Autodesk Inventor part; units mm, degrees
ref_plane "YZ Plane" through (0, 0, 0) normal (1, 0, 0) x (0, 1, 0)
ref_plane "XZ Plane" through (0, 0, 0) normal (0, 1, 0) x (-1, 0, 0)
ref_plane "XY Plane" through (0, 0, 0) normal (0, 0, 1) x (1, 0, 0)
sketch "Sketch1" plane through (0, 0, 0) normal (0, 0, 1) x (1, 0, 0)
  line L0 (-6.25, 6.25) -> (6.25, 6.25)
  line L1 (6.25, 6.25) -> (6.25, -6.25)
  line L2 (6.25, -6.25) -> (-6.25, -6.25)
  line L3 (-6.25, -6.25) -> (-6.25, 6.25)
  line L4 (-10, 10) -> (10, 10)
  line L5 (10, 10) -> (10, -10)
  line L6 (10, -10) -> (-10, -10)
  line L7 (-10, -10) -> (-10, 10)
  line L8 (-10, 10) -> (10, -10) construction
  line L9 (10, 10) -> (-10, -10) construction
  dimension "d3" = 20
  dimension "d4" = 20
  dimension "d5" = 3.75
  dimension "d6" = 16.25
  dimension "d7" = 3.75
  dimension "d8" = 16.25
extrude "Extrusion1" add sketch "Sketch1" along normal blind 55
sketch "Sketch2" plane through (0, 0, 55) normal (0, 0, 1) x (1, 0, 0)
  line L0 (10, 10) -> (-10, 10)
  line L1 (-10, -10) -> (10, -10)
  line L2 (10, -10) -> (10, 10)
  line L3 (10, 10) -> (-10, 10)
  line L4 (-10, 10) -> (-10, -10)
  line L5 (-10, -10) -> (10, 10) construction
  line L6 (10, -10) -> (-10, 10) construction
  point P0 (0, 0)
extrude "Extrusion2" add sketch "Sketch2" along normal blind 3
sketch "Sketch3" plane through (0, 0, 55) normal (0, 0, -1) x (-1, 0, 0)
  circle A0 centre (0, 0) radius 4
  dimension "d13" = 8
extrude "Extrusion3" add sketch "Sketch3" along normal blind 14
sketch "Sketch4" plane through (10, -10, 0) normal (1, 0, 0) x (0, 0, -1)
  line L0 (0, 0) -> (-58, 0)
  line L1 (0, 0) -> (-10, 0)
  line L2 (-10, 0) -> (-10, 3)
  line L3 (-10, 3) -> (0, 3)
  line L4 (0, 3) -> (0, 0)
  line L5 (-58, 0) -> (-58, 20)
  line L6 (-58, 0) -> (-48, 0)
  line L7 (-48, 0) -> (-48, 3)
  line L8 (-48, 3) -> (-58, 3)
  line L9 (-58, 3) -> (-58, 0)
  point P0 (0, 10)
  dimension "d16" = 10
  dimension "d17" = 3
  dimension "d18" = 10
  dimension "d19" = 3
extrude "Extrusion4" add sketch "Sketch4" along normal blind 10
sketch "Sketch5" plane through (-10, -10, 0) normal (-1, 0, 0) x (0, 0, 1)
  line L0 (0, 0) -> (0, 20)
  line L1 (0, 3) -> (10, 3)
  line L2 (0, 0) -> (10, 0)
  line L3 (10, 0) -> (10, 3)
  line L4 (10, 3) -> (0, 3)
  line L5 (0, 3) -> (0, 0)
  line L6 (58, 20) -> (58, 0)
  line L7 (58, 0) -> (48, 0)
  line L8 (48, 0) -> (48, 3)
  line L9 (48, 3) -> (58, 3)
  line L10 (58, 3) -> (58, 0)
  point P0 (0, 10)
  dimension "d22" = 10
  dimension "d23" = 3
  dimension "d24" = 10
  dimension "d25" = 3
extrude "Extrusion5" add sketch "Sketch5" along normal blind 10
fillet "Fillet1" radius 5 12 edges at (-20, -8.5, 10) (-20, -8.5, 0) (-10, -8.5, 10) (-10, -8.5, 48) (-20, -8.5, 48) (-20, -8.5, 58) (20, -8.5, 0) (10, -8.5, 10) (20, -8.5, 10) (10, -8.5, 48) (20, -8.5, 48) (20, -8.5, 58)
sketch "Sketch6" plane through (10, -7, 15) normal (0, 1, 0) x (1, 0, 0)
  arc A0 (-25, 15) -> (-25, 5) centre (-25, 10) ccw
  circle A1 centre (-25, 10) radius 2
  arc A2 (5, 5) -> (5, 15) centre (5, 10) ccw
  circle A3 centre (5, 10) radius 2
  arc A4 (-25, -33) -> (-25, -43) centre (-25, -38) ccw
  circle A5 centre (-25, -38) radius 2
  arc A6 (5, -43) -> (5, -33) centre (5, -38) ccw
  circle A7 centre (5, -38) radius 2
  point P0 (-10, 15)
  dimension "d29" = 4
  dimension "d30" = 4
  dimension "d31" = 4
extrude "Extrusion6" cut sketch "Sketch6" against normal blind 10
fillet "Fillet2" radius 5 2 edges at (-10, 10, 29) (10, 10, 29)
sketch "Sketch7" plane through (-5, 10, 0) normal (0, 1, 0) x (1, 0, 0)
  arc A0 (7.7, -10) -> (2.3, -10) centre (5, -10) ccw
  line L0 (0, -58) -> (0, 0)
  arc A1 (2.3, -14.35) -> (7.7, -14.35) centre (5, -14.35) ccw
  line L1 (2.3, -14.35) -> (2.3, -10)
  line L2 (7.7, -14.35) -> (7.7, -10)
  point P0 (5, 0)
  dimension "d35" = 5.4
  dimension "d36" = 5
  dimension "d37" = 10
  dimension "d38" = 5.4
  dimension "d39" = 4.35
  dimension "d40" = 5
extrude "Extrusion7" cut sketch "Sketch7" against normal blind 10
sketch "Sketch8" plane through (-5, 10, 0) normal (0, 1, 0) x (1, 0, 0)
  line L0 (2.3, -10) -> (2.3, -14.35)
  line L1 (2.3, -12.175) -> (-5, -12.175)
  line L2 (-5, 0) -> (-5, -58)
  arc A0 (-5, -15) -> (-10, -10) centre (-10, -15) ccw
  line L3 (-5, -12.175) -> (-5, -15)
  line L4 (-5, -15) -> (-18.139, -15)
  line L5 (-18.139, -15) -> (-18.139, 3.699)
  line L6 (-18.139, 3.699) -> (27.6458, 3.699)
  line L7 (27.6458, 3.699) -> (27.6458, -15)
  line L8 (15, -15) -> (15, -43)
  line L9 (27.6458, -15) -> (15, -15)
  line L10 (15, -15) -> (15, -12.175)
  arc A1 (20, -10) -> (15, -15) centre (20, -15) ccw
  line L11 (15, -12.175) -> (2.3, -12.175)
  point P0 (5, 0)
  dimension "d43" = 12.6458
  dimension "d44" = 33.139
  dimension "d45" = 18.699
extrude "Extrusion8" cut sketch "Sketch8" against normal blind 20
sketch "Sketch9" plane through (-2.7, 10, 12.175) normal (0, 0, -1) x (-1, 0, 0)
  circle A0 centre (-10.825, -10) radius 0.925
  circle A1 centre (-2.7, -18.125) radius 0.925
  circle A2 centre (5.425, -10) radius 0.925
  line L0 (-12.7, -20) -> (-12.7, -5)
  line L1 (7.3, -20) -> (-12.7, -20)
  line L2 (3.55, -16.25) -> (3.55, -3.75)
  point P0 (-2.7, -10)
  dimension "d48" = 1.85
  dimension "d49" = 1.85
  dimension "d50" = 1.85
  dimension "d51" = 1.875
  dimension "d52" = 1.875
  dimension "d53" = 1.875
  dimension "d54" = 0
  dimension "d55" = 0
  dimension "d56" = 0
extrude "Extrusion9" cut sketch "Sketch9" against normal blind 5
properties part number "14 slot pinhuls groot"
The model under review builds one solid part; all positions refer to its coordinate system, in mm. A direction names the side the tool comes from. Round coordinates to 2 decimals unless told otherwise and drop trailing zeros. Loops run counter-clockwise (first coordinate to the right, second up) from the corner with the lowest first, then second, coordinate; pieces in that order, holes last. Notation, with made-up numbers: (-24, -39.75) -> (-1, -39.75) arc R20 cw to (-1, -13.75) -> close; hole circle Ø7 at (56.25, -39). An arc over 180 degrees is marked (long way). Return JSON: item names as keys, results as strings.
(1) For faces 4 (the flat face through (10, -2, 35)), 5 (the flat face through (2.7, 8, 13)), 6 (the cylindrical face through (-8, 9, 35)), 7 (the flat face through (0, -8, 17.175)), list the 3-axis set-ups (+Z, -Z, +X, -X, +Y, -Y) from which the entire face can be reached by the end or side of a thin tool; tool diameter is ignored.
Solved:
{"face 4": "-Z, +X, +Y", "face 5": "-Z, +Y", "face 6": "+Z, -Z, -X, +Y", "face 7": "-Z"}
(2) For pin 1 (5 mm diameter, centred on x = 17, z = 52.5, fed in from +Y); pin 2 (1 mm diameter, centred on y = 3.5, z = 24.5, fed in from -X); pin 3 (2.5 mm diameter, centred on y = 8.5, z = 13, fed in from +X), all flat-tipped, find the tip position at first contact; note any pin that passes through.
Solved:
{"pin 1": "y = -7", "pin 2": "x = -10", "pin 3": "x = 9.47"}
(3) The part is to be moulded in two halves that separate along Y. For faces 1 (the flat face through (13, -7, 52)), 2 (the flat face through (0, 6.25, 33)), 3 (the flat face through (-10, -3, 35)), say which applies: released by +Y, released by -Y, zero draft, split by the parting line, or undercut.
Solved:
{"face 1": "released by +Y", "face 2": "undercut", "face 3": "zero draft"}
(4) Add section A-A on z = 34.5. Write out the cut boundary in (x, y), plus the area to 3 significant figures.
Solved:
{"outline": "(-10, -10) -> (10, -10) -> (10, 5) arc R5 ccw to (5, 10) -> (-5, 10) arc R5 ccw to (-10, 5) -> close; hole (-6.25, -6.25) -> (6.25, -6.25) -> (6.25, 6.25) -> (-6.25, 6.25) -> close", "area": "233 mm2"}
(5) Add section D-D on y = -3. Write out the cut boundary in (x, z) (3 decimals), plus the area to 3 significant figures.
Solved:
{"outline": "(-10, 12.175) -> (-6.25, 12.175) -> (-6.25, 55) -> (-2.646, 55) -> (-2.646, 41) -> (2.646, 41) -> (2.646, 55) -> (6.25, 55) -> (6.25, 12.175) -> (10, 12.175) -> (10, 58) -> (-10, 58) -> close", "area": "455 mm2"}
(6) For line 1 (X direction, y = -8.3, z = 53); line 2 (X direction, y = -3.5, z = 22), list the stretches that pass through material, from the lowest coordinate up.
Solved:
{"line 1": "-20 to -17, -13 to 13, 17 to 20", "line 2": "-10 to -6.25, 6.25 to 10"}
(7) Add section B-B on x = 0. Write out the cut boundary in (y, z) (3 decimals), plus the area to 3 significant figures.
Solved:
{"outline": "(-10, 12.175) -> (-9.05, 12.175) -> (-9.05, 17.175) -> (-7.2, 17.175) -> (-7.2, 12.175) -> (-6.25, 12.175) -> (-6.25, 55) -> (-4, 55) -> (-4, 41) -> (4, 41) -> (4, 55) -> (6.25, 55) -> (6.25, 17.05) -> (10, 17.05) -> (10, 58) -> (-10, 58) -> close", "area": "466 mm2"}
(8) Add section C-C on y = 0. Write out the cut boundary in (x, z) (3 decimals), plus the area to 3 significant figures.
Solved:
{"outline": "(-10, 12.175) -> (-9.05, 12.175) -> (-9.05, 17.175) -> (-7.2, 17.175) -> (-7.2, 12.175) -> (-6.25, 12.175) -> (-6.25, 55) -> (-4, 55) -> (-4, 41) -> (4, 41) -> (4, 55) -> (6.25, 55) -> (6.25, 12.175) -> (7.2, 12.175) -> (7.2, 17.175) -> (9.05, 17.175) -> (9.05, 12.175) -> (10, 12.175) -> (10, 58) -> (-10, 58) -> close", "area": "475 mm2"}
